Check sheet for the modelled part. Datum: model origin and axes. Units: mm. Face numbers are marked on the shaded views. A direction names the side the tool comes from. Give positions to 0.01 mm unless a question says otherwise; leave off trailing zeros. Order: outer loops, then holes, each group sorted by start corner. A loop starts at its lowest first (then second) coordinate and runs counter-clockwise, first axis right, second up. Notation, with made-up numbers: (-19.75, 16.25) - (8.25, 16.25) arc R34 ccw to (8.25, 47.25) - close; hole circle Ø10 at (86.5, 8.25). An arc over 180 degrees is marked (long way). Answer in a Markdown table with one row per item.
from build123d import *

# Parameters (mm, degrees)
SKETCH2_R           = 49.784
BOSS_EXTRUDE1_DEPTH = 203.2
SKETCH3_R           = 11.74839717
BOSS_EXTRUDE2_DEPTH = 50.8
SKETCH4_R           = 54.60446946
CUT_EXTRUDE1_DEPTH  = 382


with BuildPart() as part:
    # Sketch1 → Revolve1 (revolve)
    with BuildSketch(Plane.XY):
        with BuildLine():
            Line((304.8, 49.784), (304.8, 0))
            Line((304.8, 0), (0, 0))
            Line((0, 0), (0, 11.748397173))
            add(Edge.make_bspline(
                [(0, 11.748397173), (0.424160675, 11.855932678), (1.277768006, 12.07173392), (3.085410505, 12.527272667), (5.106222596, 13.032281093), (7.110128552, 13.529344024), (9.159948224, 14.034387922), (11.195444228, 14.532141119), (13.233412884, 15.026861964), (15.805049223, 15.64653599), (18.91026091, 16.387291474), (22.550652523, 17.244690048), (26.727238439, 18.213147263), (31.952168035, 19.405675489), (42.412897925, 21.742539102), (62.333903875, 25.976370199), (110.770450737, 35.225121195), (160.70732909, 42.159920913), (207.702302928, 46.434962608), (245.168015054, 48.368183749), (253.734807707, 48.740972714), (260.161369668, 48.98354131), (264.446272339, 49.130442523), (268.731666265, 49.262530797), (273.017475857, 49.379804553), (277.303691578, 49.48226239), (281.590188304, 49.569903083), (285.329649653, 49.633426545), (288.521672796, 49.67849525), (291.166731437, 49.70980578), (293.263778354, 49.731088433), (295.359186858, 49.74882407), (297.470177021, 49.76301264), (299.535126271, 49.773654103), (301.617177871, 49.780748429), (303.482211221, 49.783408805), (304.362420109, 49.784), (304.8, 49.784)],
                knots=[0.082917815, 0.082917815, 0.082917815, 0.082917815, 0.082917815, 0.088601511, 0.094285207, 0.099968902, 0.105652598, 0.111336294, 0.11701999, 0.122703686, 0.128387381, 0.140005218, 0.151623054, 0.16324089, 0.174858727, 0.198094396, 0.267801409, 0.383979763, 0.709279153, 0.744132659, 0.778986165, 0.790604, 0.802221836, 0.813839671, 0.825457507, 0.837075342, 0.848693177, 0.860311013, 0.871928848, 0.877612544, 0.883296239, 0.888979935, 0.89466363, 0.900347326, 0.906031021, 0.911714717, 0.917398412, 0.917398412, 0.917398412, 0.917398412, 0.917398412], degree=4))
        make_face()
    revolve(axis=Axis((304.8, 0, 0), (-1, 0, 0)))

    # Sketch2 → Boss-Extrude1 (add)
    with BuildSketch(Plane(origin=(304.8, 0, 0), x_dir=(0, 0, -1), z_dir=(1, 0, 0))):
        Circle(SKETCH2_R)
    extrude(amount=BOSS_EXTRUDE1_DEPTH)

    # Sketch3 → Boss-Extrude2 (add)
    with BuildSketch(Plane.ZY):
        Circle(SKETCH3_R)
    extrude(amount=BOSS_EXTRUDE2_DEPTH)

    # Sketch4 → Cut-Extrude1 (cut, through all)
    with BuildSketch(Plane(origin=(127, 0, 0), x_dir=(0, 0, -1), z_dir=(1, 0, 0))):
        Circle(SKETCH4_R)
    extrude(amount=CUT_EXTRUDE1_DEPTH, mode=Mode.SUBTRACT)


solid = part.part
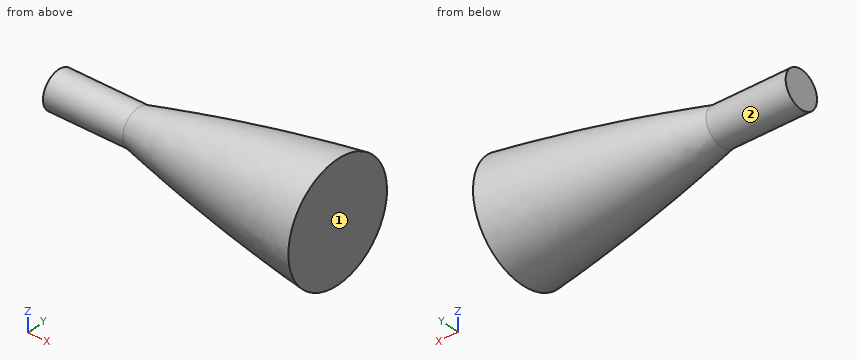
(1) Cross-section at A-A, the plane x = -15. Record the cut outline in (y, z), then the cut area to 3 significant figures.
Geometry says:
| item | result |
|---|---|
| outline | circle Ø23.5 at (0, 0) |
| area | 434 mm² |
(2) Gauge pin test, flat ends, axial feed: P1, Ø5, axis at x = -12.5, y = -4.5, coming from the +Z side; P2, Ø12, axis at x = 68.5, y = -8.5, coming from the -Z side; P3, Ø10, axis at x = -17.5, z = -8.5, coming from the +Y side. Record the tip position at first contact, or that the pin passes through.
Geometry says:
| item | result |
|---|---|
| P1 | z = 11.58 |
| P2 | z = -27.56 |
| P3 | y = 11.21 |
(3) Access from +Z, -Z, +X, -X, +Y, -Y to the whole of each face (thin tool, end or side, straight path). Record for the marked faces 1 and 2.
Geometry says:
| item | result |
|---|---|
| face 1 | +Z, -Z, +X, +Y, -Y |
| face 2 | -X |
(4) Thickness scan on L1, parallel to Y at x = 100, z = 18; L2, parallel to Y at x = 27.5, z = 7; L3, parallel to Z at x = 41.5, y = 16. Record the ranges inside material, lowest first.
Geometry says:
| item | result |
|---|---|
| L1 | -27.37 to 27.37 |
| L2 | -17 to 17 |
| L3 | -14.38 to 14.38 |
